Here's the drawing with two shaded views (mm, measured from the low corner). I have some questions. Round coordinates to 2 decimals unless told otherwise and drop trailing zeros. Loops run counter-clockwise (first coordinate to the right, second up) from the corner with the lowest first, then second, coordinate; pieces in that order, holes last. Notation, with made-up numbers: M 32,14.25 L 85,14.25 A18 cw 85,36.25 Z; hole C -33,48 d11. An arc over 180 degrees is marked long. One line per item, written item: value. Start each with the question number.
Q1. Thinking about a two-plate mould opening in Z: for the marked faces 1, 2 and 3, which applies, released by +Z, released by -Z, zero draft, split by the parting line, or undercut?
Q2. Please list where these lines run through material, in increasing order: line 1 along X through (y, z) = (2.15, 7); line 2 along X through (y, z) = (1.3, 5.5); line 3 along X through (y, z) = (3, 2.75).
Q3. Imagine slicing it at B-B (x = 30). Please give me the cut outline in (y, z) (1 decimal).
Q4. Imagine slicing it at D-D (z = 6.25). Give the number of separate pieces and of enclosed holes in the cut face, then the cut area to 3 significant figures.
Q5. I'm going to push flat-ended pins straight in: pin 1 Ø4.5 at (x, z) = (30, 7) entering from +Y; pin 2 Ø3 at (x, z) = (12, 7) entering from -Y; pin 3 Ø2 at (x, y) = (46, 4) entering from -Z; pin 4 Ø2 at (x, y) = (45, 3.5) entering from +Z. Where does each tip first touch, or does it pass through?
Q6. Imagine slicing it at C-C (x = 42.5). Please give me the cut outline in (y, z).
Q7. Imagine slicing it at A-A (y = 0.5). Please give me the cut outline in (x, z).
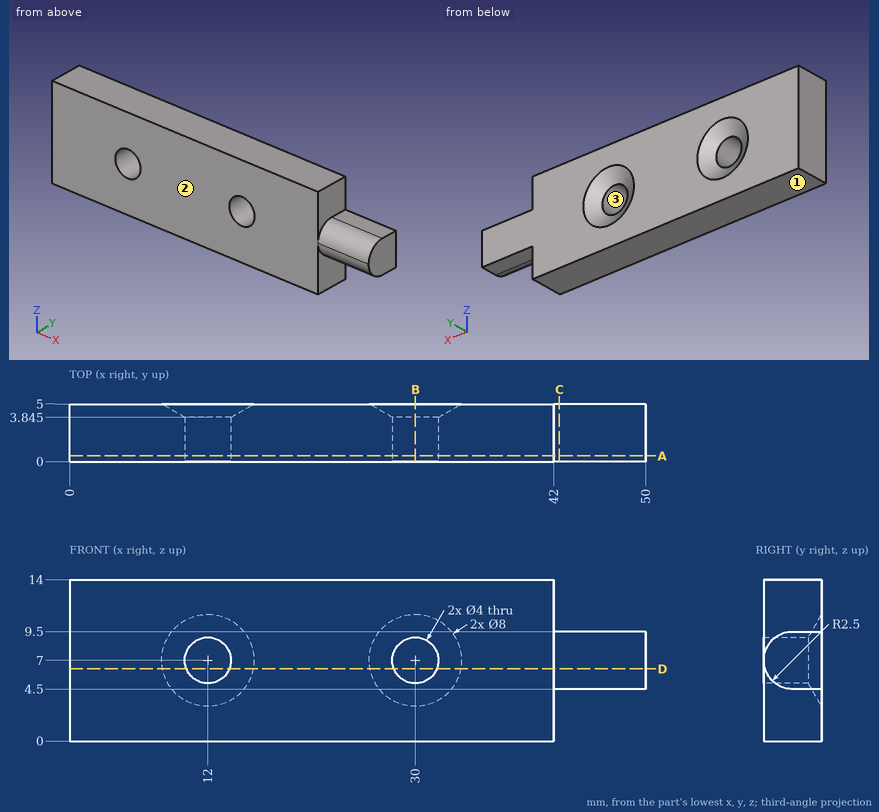
Report:
1. face 1: released by -Z
1. face 2: zero draft
1. face 3: undercut
2. line 1: x = 0 to 10, 14 to 28, 32 to 50
2. line 2: x = 0 to 10.68, 13.32 to 28.68, 31.32 to 50
2. line 3: x = 0 to 42
3. outline: M 0,0 L 5,0 L 5,3 L 3.8,5 L 0,5 Z; M 0,9 L 3.8,9 L 5,11 L 5,14 L 0,14 Z
4. separate pieces: 3
4. enclosed holes: 0
4. area: 207 mm²
5. pin 1: stops at y = 3.99
5. pin 2: passes through
5. pin 3: stops at z = 4.5
5. pin 4: stops at z = 9.5
6. outline: M 2.5,4.5 L 5,4.5 L 5,9.5 L 2.5,9.5 A2.5 ccw Z
7. outline: M 0,0 L 42,0 L 42,5.5 L 50,5.5 L 50,8.5 L 42,8.5 L 42,14 L 0,14 Z; hole C 12,7 d4; hole C 30,7 d4
